from build123d import *

# Parameters (mm, degrees)
CROQUIS1_R                                           = 2.55
SALIENTE_EXTRUIR1_DEPTH                              = 3
AVELLANADO_PARA_TORNILLO_CON_CABEZA_AVEL_D           = 5.5
AVELLANADO_PARA_TORNILLO_CON_CABEZA_AVEL_DEPTH       = 5
AVELLANADO_PARA_TORNILLO_CON_CABEZA_AVEL_CSINK_D     = 11.47
AVELLANADO_PARA_TORNILLO_CON_CABEZA_AVEL_CSINK_ANGLE = 90
AVELLANADO_PARA_TORNILLO_CON_CABEZA_AVEL_TIP         = 1.652366702


with BuildPart() as part:
    # Croquis1 → Saliente-Extruir1 (new body)
    with BuildSketch(Plane.XY):
        with BuildLine():
            Line((2, 0), (38, 0))
            ThreePointArc((38, 0), (39.414213562, 0.585786438), (40, 2))
            Line((40, 2), (40, 18))
            ThreePointArc((40, 18), (39.414213562, 19.414213562), (38, 20))
            Line((38, 20), (2, 20))
            ThreePointArc((2, 20), (0.585786438, 19.414213562), (0, 18))
            Line((0, 18), (0, 2))
            ThreePointArc((0, 2), (0.585786438, 0.585786438), (2, 0))
        make_face()
        with Locations((10, 10)):
            Circle(CROQUIS1_R, mode=Mode.SUBTRACT)
        with Locations((20, 10)):
            Circle(CROQUIS1_R, mode=Mode.SUBTRACT)
        with Locations((30, 10)):
            Circle(CROQUIS1_R, mode=Mode.SUBTRACT)
    extrude(amount=SALIENTE_EXTRUIR1_DEPTH)

    # Avellanado para tornillo con cabeza avellanada de clavija hexagonal de M51
    with Locations(Plane.XY.offset(3)):
        with Locations((10, 10), (30, 10)):
            CounterSinkHole(AVELLANADO_PARA_TORNILLO_CON_CABEZA_AVEL_D / 2, AVELLANADO_PARA_TORNILLO_CON_CABEZA_AVEL_CSINK_D / 2, depth=AVELLANADO_PARA_TORNILLO_CON_CABEZA_AVEL_DEPTH, counter_sink_angle=AVELLANADO_PARA_TORNILLO_CON_CABEZA_AVEL_CSINK_ANGLE)
            with Locations((0, 0, -(AVELLANADO_PARA_TORNILLO_CON_CABEZA_AVEL_DEPTH + AVELLANADO_PARA_TORNILLO_CON_CABEZA_AVEL_TIP / 2))):  # 118° drill point
                Cone(0, AVELLANADO_PARA_TORNILLO_CON_CABEZA_AVEL_D / 2, AVELLANADO_PARA_TORNILLO_CON_CABEZA_AVEL_TIP, mode=Mode.SUBTRACT)


solid = part.part
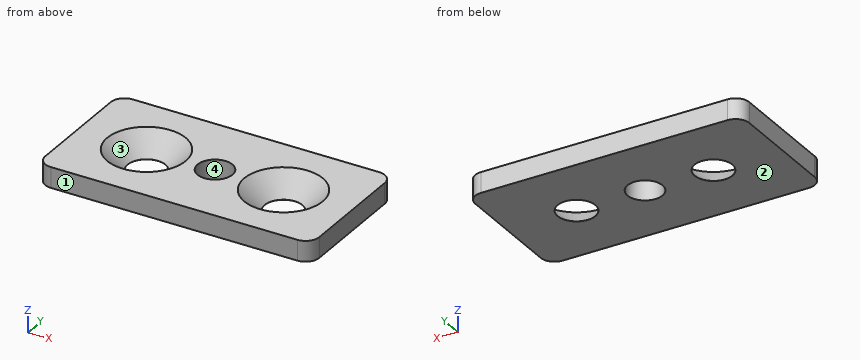
The model under review builds one solid part; all positions refer to its coordinate system, in mm. Face numbers are marked on the shaded views. Coordinates: 2 decimals unless noted, no trailing zeros. Write each loop counter-clockwise with the first axis right and the second up, starting at its lowest first coordinate (ties: lowest second). Pieces come first, ordered by that corner, then holes. Notation, with made-up numbers: (-19.75, 60) -> (30.25, 60) arc R26 ccw to (30.25, 91) -> close; hole circle Ø2 at (-16.75, -14.75). An arc over 180 degrees is marked (long way). Answer in a Markdown table with one row per item.
1. Draft analysis for pull direction Y (two halves, no side actions). For the marked faces 1, 2, 3 and 4, state which applies: +Y half, -Y half, draft (parallel to the pull), parting line (faces both ways), or undercut.
Answers below:
| item | result |
|---|---|
| face 1 | -Y half |
| face 2 | draft |
| face 3 | undercut |
| face 4 | undercut |
2. Clearance check with flat-ended pins moving along their axes: pin 1 Ø4 at (x, y) = (12, 11.5) entering from +Z (3 decimals); pin 2 Ø3.5 at (x, y) = (10, 10) entering from -Z. State where each tip first meets the part, or that it passes through.
Answers below:
| item | result |
|---|---|
| pin 1 | stops at z = 1.765 |
| pin 2 | passes through |
3. We need section C-C, the plane z = 1.45. State the section outline as (x, y) points (3 decimals), and give its area (3 significant figures).
Answers below:
| item | result |
|---|---|
| outline | (0, 2) arc R2 ccw to (2, 0) -> (38, 0) arc R2 ccw to (40, 2) -> (40, 18) arc R2 ccw to (38, 20) -> (2, 20) arc R2 ccw to (0, 18) -> close; hole circle Ø8.37 at (10, 10); hole circle Ø5.1 at (20, 10); hole circle Ø8.37 at (30, 10) |
| area | 666 mm^2 |
4. We need section B-B, the plane y = 10. State the section outline as (x, z) points (3 decimals), and give its area (3 significant figures).
Answers below:
| item | result |
|---|---|
| outline | (0, 0) -> (7.25, 0) -> (7.25, 0.015) -> (4.265, 3) -> (0, 3) -> close; (12.75, 0) -> (17.45, 0) -> (17.45, 3) -> (15.735, 3) -> (12.75, 0.015) -> close; (22.55, 0) -> (27.25, 0) -> (27.25, 0.015) -> (24.265, 3) -> (22.55, 3) -> close; (32.75, 0) -> (40, 0) -> (40, 3) -> (35.735, 3) -> (32.75, 0.015) -> close |
| area | 53.9 mm^2 |
5. Wall thickness on probe 1 along X at (y, z) = (10.75, 0.8); probe 2 along X at (y, z) = (9.25, 1.85); probe 3 along Y at (x, z) = (30.5, 2.5): over which ranges is each line inside the solid? List them lowest first. Write a range as [from, to].
Answers below:
| item | result |
|---|---|
| probe 1 | x = [0, 6.55], [13.45, 17.56], [22.44, 26.55], [33.45, 40] |
| probe 2 | x = [0, 5.48], [14.52, 17.56], [22.44, 25.48], [34.52, 40] |
| probe 3 | y = [0, 4.79], [15.21, 20] |
6. We need section D-D, the plane x = 10. State the section outline as (y, z) points (3 decimals).
Answers below:
| item | result |
|---|---|
| outline | (0, 0) -> (7.25, 0) -> (7.25, 0.015) -> (4.265, 3) -> (0, 3) -> close; (12.75, 0) -> (20, 0) -> (20, 3) -> (15.735, 3) -> (12.75, 0.015) -> close |
7. We need section A-A, the plane x = 20. State the section outline as (y, z) points, and give its area (3 significant figures).
Answers below:
| item | result |
|---|---|
| outline | (0, 0) -> (7.45, 0) -> (7.45, 3) -> (0, 3) -> close; (12.55, 0) -> (20, 0) -> (20, 3) -> (12.55, 3) -> close |
| area | 44.7 mm^2 |
